Source: CAD feature listing. Evaluate the final solid. Frame: model axes, mm. A direction names the side the tool comes from. Coordinates: 2 decimals unless noted, no trailing zeros. Write each loop counter-clockwise with the first axis right and the second up, starting at its lowest first coordinate (ties: lowest second). Pieces come first, ordered by that corner, then holes. Notation, with made-up numbers: M 34.5,47 L 83.5,47 A34 cw 83.5,81 Z; hole C 4,-13 d9. An arc over 180 degrees is marked long. Answer as CSV lines item,"result". Start each with the question number.
1. Section C-C on x = 0.75. Return the cut outline in (y, z).
2. Section D-D on y = -0.75. Return the cut outline in (x, z) (3 decimals), plus the area to 3 significant figures.
3. Contact query for a flat-ended pin moving along its axis: pin 1 Ø1.5 at (x, z) = (-2, 4.5) entering from -Y. Output: stop coordinate, or through.
4. Section A-A on z = 10.16. Return the cut outline in (x, y) (3 decimals), plus the area to 3 significant figures.
5. Mould query, pull axis Z, two halves, no side actions, for faces 3 (the face through (0, -5, 0)), 4 (the face through (0, -10.16, 8)), 5 (the face through (-8, -5.2, 9.4)), 6 (the face through (0, -8, 2.54)). Classes: pulls with the +Z half, pulls with the -Z half, needs draft (parallel to the pull), parting line crosses it, or undercut.
6. Reachability of faces 1 (the face through (0, -5, 12.7)), 2 (the face through (0, -5.08, 5)) from +Z, -Z, +X, -X, +Y, -Y: full face, straight path, thin tool, end or side. Return the list, or none.
7. Line query: probe 1 along X at (y, z) = (-6.5, 9) (3 decimals); probe 2 along X at (y, z) = (-7.5, 5.75) (3 decimals); probe 3 along Z at (x, y) = (-3, -6.5). Output: solid intervals per line, ascending. Write a range as [from, to].
8. Section B-B on y = -6. Return the cut outline in (x, z) (3 decimals), plus the area to 3 significant figures.
```python
from build123d import *

# Parameters (mm, degrees)
F0_W     = 19.05
F0_H     = 12.7
F1_DEPTH = 10.16
F2_W     = 12.7
F2_H     = 5.08
F3_DEPTH = 5.08
F4_R     = 1.27
F5_DEPTH = 10.16


with BuildPart() as f1:
    # F0 (on Front) → F1 (new body)
    with BuildSketch(Plane.XZ):
        with Locations((0, 6.35)):
            Rectangle(F0_W, F0_H)
    extrude(amount=F1_DEPTH)

    # F2 (on face) → F3 (cut)
    with BuildSketch(Plane.XZ.offset(10.16)):
        with Locations((0, 5.08)):
            Rectangle(F2_W, F2_H)
    extrude(amount=-F3_DEPTH, mode=Mode.SUBTRACT)

    # F4 (on face) → F5 (cut)
    with BuildSketch(Plane.XZ.offset(10.16)):
        with Locations((6.985, 10.16)):
            Circle(F4_R)
        with Locations((-6.985, 10.16)):
            Circle(F4_R)
    extrude(amount=-F5_DEPTH, mode=Mode.SUBTRACT)


solid = f1.part
```
Values:
1,outline,"M -10.16,0 L 0,0 L 0,12.7 L -10.16,12.7 L -10.16,7.62 L -5.08,7.62 L -5.08,2.54 L -10.16,2.54 Z"
2,outline,"M -9.525,0 L 9.525,0 L 9.525,12.7 L -9.525,12.7 Z; hole C -6.985,10.16 d2.54; hole C 6.985,10.16 d2.54"
2,area,"232 mm²"
3,pin 1,"y = -5.08"
4,outline,"M -9.525,-10.16 L -8.255,-10.16 L -8.255,0 L -9.525,0 Z; M -5.715,-10.16 L 5.715,-10.16 L 5.715,0 L -5.715,0 Z; M 8.255,-10.16 L 9.525,-10.16 L 9.525,0 L 8.255,0 Z"
4,area,"142 mm²"
5,face 3,"pulls with the -Z half"
5,face 4,"needs draft"
5,face 5,"undercut"
5,face 6,"undercut"
6,face 1,"+Z, +X, -X, +Y, -Y"
6,face 2,"-Y"
7,probe 1,"[-9.525, -7.502], [-6.468, 6.468], [7.502, 9.525]"
7,probe 2,"[-9.525, -6.35], [6.35, 9.525]"
7,probe 3,"[0, 2.54], [7.62, 12.7]"
8,outline,"M -9.525,0 L 9.525,0 L 9.525,12.7 L -9.525,12.7 Z; hole C -6.985,10.16 d2.54; hole M -6.35,2.54 L 6.35,2.54 L 6.35,7.62 L -6.35,7.62 Z; hole C 6.985,10.16 d2.54"
8,area,"167 mm²"
